The listing builds one solid part. Answer for the finished solid, in the listing's coordinates (mm). Give positions to 0.01 mm unless a question says otherwise; leave off trailing zeros. Loops run counter-clockwise (first coordinate to the right, second up) from the corner with the lowest first, then second, coordinate; pieces in that order, holes last. Notation, with made-up numbers: M 71,-18 L 118,-18 A16 ccw 118,-7 Z; hole C 79,15.5 d10. An arc over 180 degrees is marked long. Use one line per item in the form item = value. Start each with the question number.
1. The part is cut by section B-B (z = 15.2). Write down the section's boundary in (x, y), and give its area (3 significant figures).
2. The part is cut by section A-A (x = 0). Write down the section's boundary in (y, z), and give its area (3 significant figures).
3. The part is cut by section D-D (z = -25). Write down the section's boundary in (x, y).
4. The mould has two halves that part along X. Classify faces 1 (the face through (7.71, 1.17, -29.43)), 2 (the face through (11.06, 1.17, 13.97)), 3 (the face through (-7.77, 1.17, -29.4)): released by +X, released by -X, zero draft, split by the parting line, or undercut.
5. Straight lines are drawn through the part: line 1 (X direction, y = 1.3, z = -15.2); line 2 (X direction, y = 0.75, z = 15.5); line 3 (X direction, y = 2.05, z = 22). For each, find the intervals that lie inside material, in ascending order. Write a range as from..to.
6. Each of these flat-tipped pins is pushed along its axis until it touches: pin 1 Ø1.9 at (x, z) = (31, 19.22) entering from -Y; pin 2 Ø4 at (x, z) = (-31, 19.22) entering from +Y; pin 3 Ø1 at (x, y) = (-7.5, 2) entering from -Z. Where does it stop, or does it pass through?
7. The part is cut by section C-C (y = 1.9). Write down the section's boundary in (x, z), and give its area (3 significant figures).
from build123d import *

# Parameters (mm, degrees)
SKETCH1_R           = 1.55
BOSS_EXTRUDE1_DEPTH = 2.38


with BuildPart() as part:
    # Sketch1 → Boss-Extrude1 (new body)
    with BuildSketch(Plane(origin=(0, 0, 0), x_dir=(1, 0, 0), z_dir=(0, 1, 0))):
        with BuildLine():
            Line((-5.394574785, 30), (5.394574785, 30))
            ThreePointArc((5.394574785, 30), (7.742669354, 29.414346146), (9.54069567, 27.794580758))
            Line((9.54069567, 27.794580758), (35.146120884, -10.194369075))
            ThreePointArc((35.146120884, -10.194369075), (35.781767687, -11.527889331), (36, -12.988949833))
            Line((36, -12.988949833), (36, -19.215381939))
            ThreePointArc((36, -19.215381939), (34.535533906, -22.750915845), (31, -24.215381939))
            Line((31, -24.215381939), (-31, -24.215381939))
            ThreePointArc((-31, -24.215381939), (-34.535533906, -22.750915845), (-36, -19.215381939))
            Line((-36, -19.215381939), (-36, -12.988949833))
            ThreePointArc((-36, -12.988949833), (-35.781767687, -11.527889331), (-35.146120884, -10.194369075))
            Line((-35.146120884, -10.194369075), (-9.54069567, 27.794580758))
            ThreePointArc((-9.54069567, 27.794580758), (-7.742669354, 29.414346146), (-5.394574785, 30))
        make_face()
        with Locations(Location((0, 25, 0), (0, 0, 270))):
            Circle(SKETCH1_R, mode=Mode.SUBTRACT)
        with Locations(Location((-31, -19.215381939, 0), (0, 0, 270))):
            Circle(SKETCH1_R, mode=Mode.SUBTRACT)
        with Locations(Location((31, -19.215381939, 0), (0, 0, 270))):
            Circle(SKETCH1_R, mode=Mode.SUBTRACT)
        with Locations(Location((12, -15.2, 0), (0, 0, 270))):
            Circle(SKETCH1_R, mode=Mode.SUBTRACT)
        with Locations(Location((-12, -15.2, 0), (0, 0, 270))):
            Circle(SKETCH1_R, mode=Mode.SUBTRACT)
        with Locations(Location((-12, 15.2, 0), (0, 0, 270))):
            Circle(SKETCH1_R, mode=Mode.SUBTRACT)
        with Locations(Location((12, 15.2, 0), (0, 0, 270))):
            Circle(SKETCH1_R, mode=Mode.SUBTRACT)
    extrude(amount=BOSS_EXTRUDE1_DEPTH)


solid = part.part
Derived:
q1.outline = M -36,0 L -13.55,0 L -13.55,2.38 L -36,2.38 Z; M -10.45,0 L 10.45,0 L 10.45,2.38 L -10.45,2.38 Z; M 13.55,0 L 36,0 L 36,2.38 L 13.55,2.38 Z
q1.area = 157 mm2
q2.outline = M 0,-30 L 2.38,-30 L 2.38,-26.55 L 0,-26.55 Z; M 0,-23.45 L 2.38,-23.45 L 2.38,24.22 L 0,24.22 Z
q2.area = 122 mm2
q3.outline = M -11.42,0 L -1.55,0 L -1.55,2.38 L -11.42,2.38 Z; M 1.55,0 L 11.42,0 L 11.42,2.38 L 1.55,2.38 Z
q4.face_1 = released by +X
q4.face_2 = undercut
q4.face_3 = released by -X
q5.line_1 = -18.03..-13.55, -10.45..10.45, 13.55..18.03
q5.line_2 = -36..-13.52, -10.48..10.48, 13.52..36
q5.line_3 = -35.15..35.15
q6.pin_1 = through
q6.pin_2 = 2.38
q6.pin_3 = -29.74
q7.outline = M -36,12.99 A5 ccw -35.15,10.19 L -9.54,-27.79 A5 ccw -5.39,-30 L 5.39,-30 A5 ccw 9.54,-27.79 L 35.15,10.19 A5 ccw 36,12.99 L 36,19.22 A5 ccw 31,24.22 L -31,24.22 A5 ccw -36,19.22 Z; hole C -31,19.22 d3.1; hole C -12,-15.2 d3.1; hole C -12,15.2 d3.1; hole C 0,-25 d3.1; hole C 12,-15.2 d3.1; hole C 12,15.2 d3.1; hole C 31,19.22 d3.1
q7.area = 2,680 mm2
